Input: part model. Units: mm. Frame: model coordinates. Face numbers are marked on the shaded views. Give positions to 0.01 mm unless a question says otherwise; leave off trailing zeros. Loops run counter-clockwise (first coordinate to the right, second up) from the corner with the lowest first, then second, coordinate; pieces in that order, holes last. Notation, with made-up numbers: (-8.75, 39) - (34.25, 39) arc R31 ccw to (34.25, 78) - close; hole circle Ø4 at (0.5, 63). An arc over 180 degrees is marked (long way). Answer as a JSON object with one key per item and string values. Group by question number.
(1) Section query A-A (y = 0). Return loops of the section in (x, z), plus the area to 3 significant figures.
(2) Section query C-C (z = 7). Return loops of the section in (x, y).
(3) Section query D-D (x = 1.5). Return loops of the section in (y, z).
(4) Material intervals for L1, parallel to Y at x = 0.55, z = 0; L2, parallel to X at y = 4.25, z = 2.5; L3, parallel to Y at x = 4.5, z = 0, sorted ascending.
(5) Pin query (flat end, axial travel): P1, Ø3, axis at x = 3, y = 2, coming from the +Z side; P2, Ø3, axis at x = 2.5, z = 6, coming from the -Y side; P3, Ø8, axis at y = -3, z = -2.5, coming from the +X side. Return the tip coordinate at first contact, or that it passes through.
(6) Mould query, pull axis Y, two halves, no side actions, for the marked faces 1, 2 and 3. Classes: +Y half, -Y half, draft (parallel to the pull), parting line (faces both ways), or undercut.
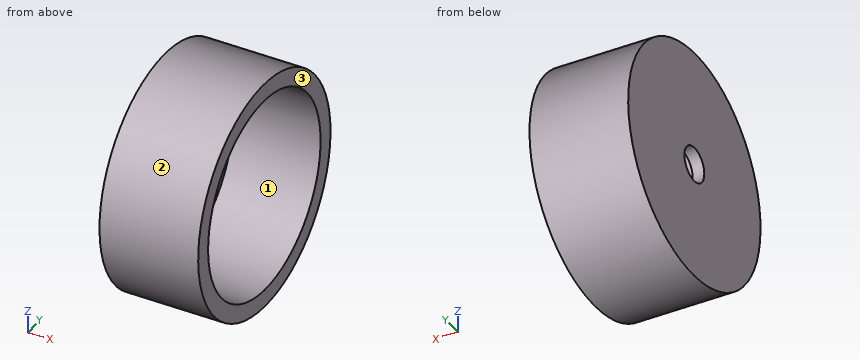
```python
from build123d import *

# Parameters (mm, degrees)
SKETCH_1_R          = 10
SKETCH_1_R_2        = 8.5
EXTRUDE_1_DEPTH     = 8.5
SKETCH_2_R          = 8.5
EXTRUDE_2_DEPTH     = 1
SKETCH_7_R          = 1.5
CUT_EXTRUDE_3_DEPTH = 17.5


with BuildPart() as part:
    # ｽｹｯﾁ1 → ﾎﾞｽ - 押し出し1 (new body)
    with BuildSketch(Plane.YZ):
        with Locations(Location((0, 0, 0), (0, 0, 270))):
            Circle(SKETCH_1_R)
        with Locations(Location((0, 0, 0), (0, 0, 270))):
            Circle(SKETCH_1_R_2, mode=Mode.SUBTRACT)
    extrude(amount=EXTRUDE_1_DEPTH)

    # ｽｹｯﾁ2 → ﾎﾞｽ - 押し出し2 (add)
    with BuildSketch(Plane(origin=(0, 0, 0), x_dir=(0, -1, 0), z_dir=(-1, 0, 0))):
        with Locations(Location((0, 0, 0), (0, 0, 90))):
            Circle(SKETCH_2_R)
    extrude(amount=-EXTRUDE_2_DEPTH)

    # ｽｹｯﾁ7 → ｶｯﾄ - 押し出し3 (cut, through all)
    with BuildSketch(Plane(origin=(0, 0, 0), x_dir=(0, -1, 0), z_dir=(-1, 0, 0))):
        with Locations(Location((0, 0, 0), (0, 0, 90))):
            Circle(SKETCH_7_R)
    extrude(amount=-CUT_EXTRUDE_3_DEPTH, mode=Mode.SUBTRACT)


solid = part.part
```
Recorded:
{
 "1": {"outline": "(0, -10) - (8.5, -10) - (8.5, -8.5) - (1, -8.5) - (1, -1.5) - (0, -1.5) - close; (0, 1.5) - (1, 1.5) - (1, 8.5) - (8.5, 8.5) - (8.5, 10) - (0, 10) - close", "area": "39.5 mm^2"},
 "2": {"outline": "(0, -7.14) - (8.5, -7.14) - (8.5, -4.82) - (1, -4.82) - (1, 4.82) - (8.5, 4.82) - (8.5, 7.14) - (0, 7.14) - close"},
 "3": {"outline": "circle Ø20 at (0, 0); hole circle Ø17 at (0, 0)"},
 "4": {"L1": "y = -10 to -1.5, 1.5 to 10", "L2": "x = 0 to 1", "L3": "y = -10 to -8.5, 8.5 to 10"},
 "5": {"P1": "stops at z = 9.99", "P2": "stops at y = -8.93", "P3": "stops at x = 1"},
 "6": {"face 1": "undercut", "face 2": "parting line", "face 3": "draft"}
}
